Study the drawing (mm; zero at the part's minimum x, y, z) and answer. Coordinates: 2 decimals unless noted, no trailing zeros. Write each loop counter-clockwise with the first axis right and the second up, starting at its lowest first coordinate (ties: lowest second). Pieces come first, ordered by that corner, then holes. Notation, with made-up numbers: (-28.75, 49.5) -> (4.25, 49.5) arc R22 ccw to (4.25, 59.5) -> close; hole circle Ø8 at (-14, 80). An arc over 180 degrees is marked (long way). Write item = value, one per line. Start each with the question number.
1) Section D-D (y = 113) is taken. Determine the outline of the cut face in (x, z), plus the area to 3 significant figures.
2) Find the intervals of material crossed by line 1 along Y through (x, z) = (80, 2.35); line 2 along X through (y, z) = (65, 2); line 3 along X through (y, z) = (65.5, 1.8), in increasing order. Write a range as from..to.
3) Flat-ended cylindrical pins translate along their axes: pin 1 Ø1.8 at (x, y) = (30, 25) entering from -Z; pin 2 Ø1.5 at (x, z) = (68, 1) entering from +Y; pin 3 Ø5 at (x, y) = (80, 25) entering from -Z. Find the tip coordinate at first contact, or state that the pin passes through.
4) Section C-C (y = 25) is taken. Determine the outline of the cut face in (x, z).
5) Section B-B (z = 1.15) is taken. Determine the outline of the cut face in (x, y).
6) Section A-A (x = 30) is taken. Determine the outline of the cut face in (y, z).
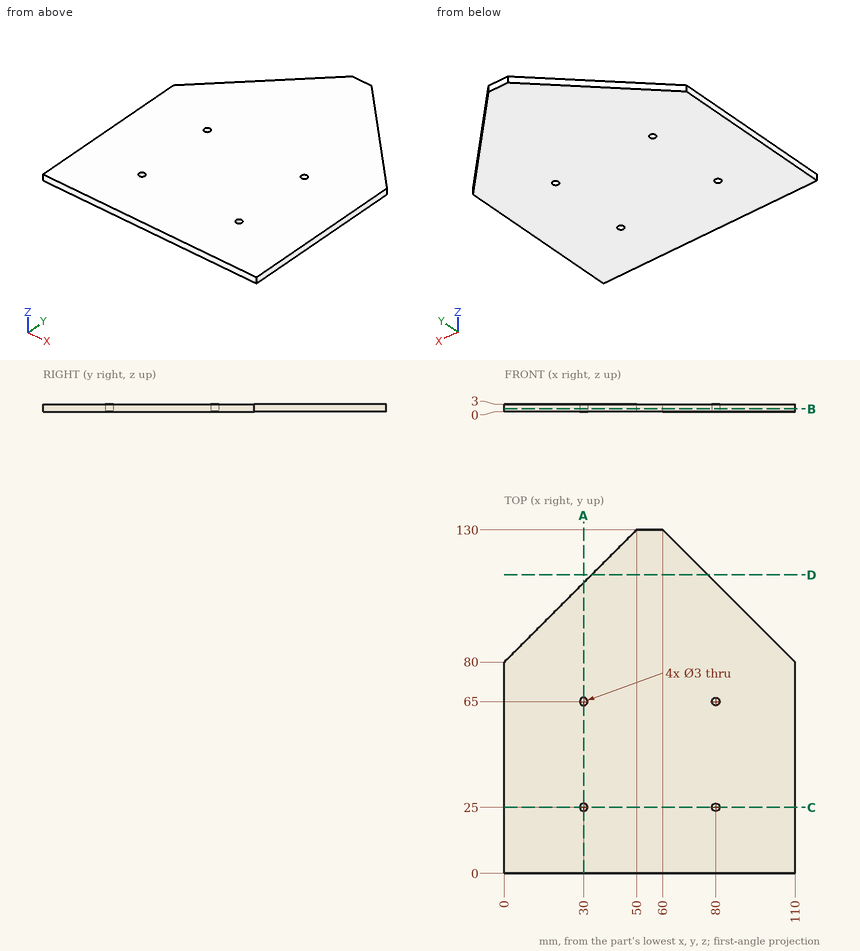
Answer key:
q1.outline = (33, 0) -> (77, 0) -> (77, 3) -> (33, 3) -> close
q1.area = 132 mm^2
q2.line_1 = 0..23.5, 26.5..63.5, 66.5..110
q2.line_2 = 0..28.5, 31.5..78.5, 81.5..110
q2.line_3 = 0..28.59, 31.41..78.59, 81.41..110
q3.pin_1 = through
q3.pin_2 = 122.75
q3.pin_3 = 0
q4.outline = (0, 0) -> (28.5, 0) -> (28.5, 3) -> (0, 3) -> close; (31.5, 0) -> (78.5, 0) -> (78.5, 3) -> (31.5, 3) -> close; (81.5, 0) -> (110, 0) -> (110, 3) -> (81.5, 3) -> close
q5.outline = (0, 0) -> (110, 0) -> (110, 80) -> (60, 130) -> (50, 130) -> (0, 80) -> close; hole circle Ø3 at (30, 25); hole circle Ø3 at (30, 65); hole circle Ø3 at (80, 25); hole circle Ø3 at (80, 65)
q6.outline = (0, 0) -> (23.5, 0) -> (23.5, 3) -> (0, 3) -> close; (26.5, 0) -> (63.5, 0) -> (63.5, 3) -> (26.5, 3) -> close; (66.5, 0) -> (110, 0) -> (110, 3) -> (66.5, 3) -> close
